```python
from build123d import *

# Parameters (mm, degrees)
F0_R      = 10.5
F1_DEPTH  = 54
F3_R      = 7.5
F1_FACE_R = 10.5
F5_W      = 9
F5_H      = 9
F6_DEPTH  = 16


with BuildPart() as f1:
    # F0 (on Top) → F1 (new body)
    with BuildSketch(Plane.XY):
        Circle(F0_R)
    extrude(amount=F1_DEPTH)

    # F3 (on offset) → F4 section 0
    with BuildSketch(Plane.XY.offset(74)):
        Circle(F3_R)
    # F1_face (on face) → F4 section 1
    with BuildSketch(Plane.XY.offset(54)):
        Circle(F1_FACE_R)
    loft()

    # F5 (on face) → F6 (cut)
    with BuildSketch(Plane.XY.offset(74)):
        Rectangle(F5_W, F5_H)
    extrude(amount=-F6_DEPTH, mode=Mode.SUBTRACT)


solid = f1.part
```
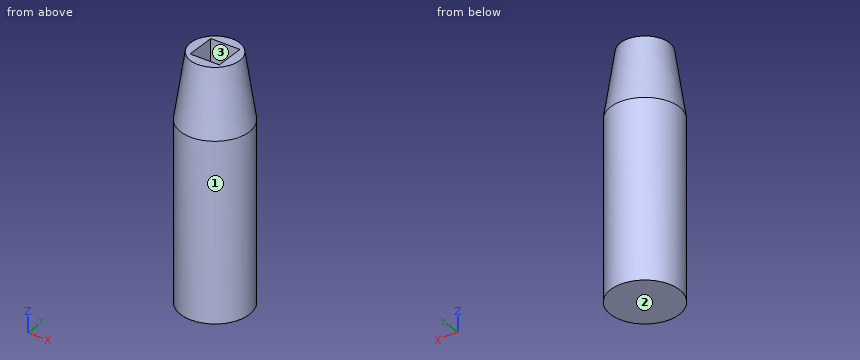
Input: part model. Units: mm. Frame: model coordinates. Face numbers are marked on the shaded views. Give positions to 0.01 mm unless a question says otherwise; leave off trailing zeros. Order: outer loops, then holes, each group sorted by start corner. A loop starts at its lowest first (then second) coordinate and runs counter-clockwise, first axis right, second up. Notation, with made-up numbers: (36.25, 70.25) -> (64.25, 70.25) arc R18 ccw to (64.25, 92.25) -> close; hole circle Ø8 at (26, 70). An arc over 180 degrees is marked (long way). Write each question's results on one line, items separated by ' | '. Start each with the question number.
Item 1: Cut plane B-B on z = 52. Return the cut outline in (x, y), then the cut area to 3 significant figures.
Item 2: Cut plane A-A on x = 0. Return the cut outline in (y, z), then the cut area to 3 significant figures.
Item 3: Mould query, pull axis Y, two halves, no side actions, for the marked faces 1, 2 and 3. Classes: pulls with the +Y half, pulls with the -Y half, needs draft (parallel to the pull), parting line crosses it, or undercut.
Item 4: Contact query for flat-ended pins moving along their axis: P1, Ø5, axis at x = 4.5, z = 22, coming from the +Y side; P2, Ø1.5, axis at x = -7, z = 34.5, coming from the -Y side; P3, Ø7, axis at y = -0.5, z = 69.5, coming from the +X side. Output: stop coordinate, or through.
Item 5: Line query: line 1 (Y direction, x = 3, z = 60); line 2 (Y direction, x = -0.5, z = 48); line 3 (X direction, y = -1.5, z = 69). Output: solid intervals per line, ascending.
Established:
1) outline: circle Ø21 at (0, 0) | area: 346 mm^2
2) outline: (-10.5, 0) -> (10.5, 0) -> (10.5, 54) -> (7.5, 74) -> (4.5, 74) -> (4.5, 58) -> (-4.5, 58) -> (-4.5, 74) -> (-7.5, 74) -> (-10.5, 54) -> close | area: 1,350 mm^2
3) face 1: parting line crosses it | face 2: needs draft | face 3: undercut
4) P1: y = 10.31 | P2: y = -8.44 | P3: x = 8.7
5) line 1: -9.12 to -4.5, 4.5 to 9.12 | line 2: -10.49 to 10.49 | line 3: -8.11 to -4.5, 4.5 to 8.11
